Check sheet for the modelled part. Datum: model origin and axes. Units: mm. Face numbers are marked on the shaded views. A direction names the side the tool comes from. Round coordinates to 2 decimals unless told otherwise and drop trailing zeros. Order: outer loops, then holes, each group sorted by start corner. A loop starts at its lowest first (then second) coordinate and runs counter-clockwise, first axis right, second up. Notation, with made-up numbers: (-4, -37) -> (44, -37) arc R23 ccw to (44, -26) -> close; hole circle Ø10 at (-38.75, 66). An arc over 180 degrees is marked (long way). Use CSV: the item, a comma, the result in double quotes.
```python
from build123d import *

# Parameters (mm, degrees)
BOSS_EXTRUDE1_DEPTH = 19.05
SKETCH2_R           = 3
CUT_EXTRUDE1_DEPTH  = 3.175
CUT_EXTRUDE2_REACH  = 48.785
SKETCH3_R           = 3
FILLET1_R           = 10


with BuildPart() as part:
    # Sketch1 → Boss-Extrude1 (new body)
    with BuildSketch(Plane(origin=(0, 0, 0), x_dir=(1, 0, 0), z_dir=(0, 1, 0))):
        Polygon((0, 0), (37.625, 0), (37.625, -6.35), (0, -6.35), (0, -9.525), (40.8, -9.525), (40.8, 3.175), (0, 3.175), align=None)
    extrude(amount=BOSS_EXTRUDE1_DEPTH)

    # Sketch2 → Cut-Extrude1 (cut)
    with BuildSketch(Plane(origin=(40.8, 0, 0), x_dir=(0, 0, -1), z_dir=(1, 0, 0))):
        with Locations((-3.175, 9.525)):
            Circle(SKETCH2_R)
    extrude(amount=-CUT_EXTRUDE1_DEPTH, mode=Mode.SUBTRACT)

    # Cut-Extrude2: up to this face of the body (flat: up to its plane)
    cut_extrude2_end = Plane(part.part.faces().sort_by_distance((20.4, 9.525, -3.175))[0])
    # Sketch3 → Cut-Extrude2 (cut, up to the picked face)
    with BuildSketch(Plane.XY.offset(9.525), mode=Mode.PRIVATE) as cut_extrude2_sk1:
        with Locations((12.7, 9.525)):
            Circle(SKETCH3_R)
    cut_extrude2_tool1 = split(extrude(cut_extrude2_sk1.sketch, amount=-CUT_EXTRUDE2_REACH, mode=Mode.PRIVATE), bisect_by=cut_extrude2_end, keep=Keep.BOTH, mode=Mode.PRIVATE)
    add(cut_extrude2_tool1.solids().sort_by(Axis((12.7, 9.525, 9.525), (0, 0, -1)))[0], mode=Mode.SUBTRACT)

    # Fillet1
    # the kernel refuses this fillet: 10 mm, written as the material it takes off along each edge
    with BuildSketch(Plane(origin=(0, 0, -28.175), x_dir=(0, 1, 0), z_dir=(0, 0, 1)), Plane(origin=(0, 19.05, -18.65), x_dir=(1, 0, 0), z_dir=(0, 0, 1))) as fillet1_piece_1:
        with BuildLine():
            CenterArc((FILLET1_R, -FILLET1_R), FILLET1_R, 90, 90)
            Line((0, -FILLET1_R), (0, 0))
            Line((0, 0), (FILLET1_R, 0))
        make_face()
    extrude(amount=53.175, mode=Mode.SUBTRACT)
    with BuildSketch(Plane(origin=(0, 19.05, -28.175), x_dir=(0, -1, 0), z_dir=(0, 0, 1)), Plane(origin=(0, 0, -18.65), x_dir=(1, 0, 0), z_dir=(0, 0, 1))) as fillet1_piece_2:
        with BuildLine():
            CenterArc((FILLET1_R, FILLET1_R), FILLET1_R, 180, 90)
            Line((0, FILLET1_R), (0, 0))
            Line((0, 0), (FILLET1_R, 0))
        make_face()
    extrude(amount=53.175, mode=Mode.SUBTRACT)


solid = part.part
```
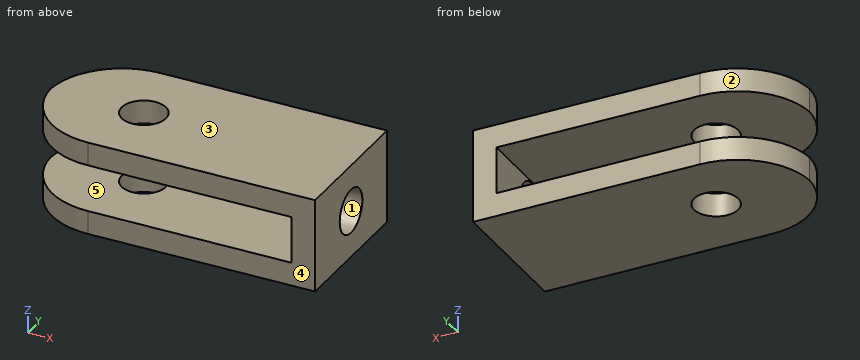
Q1. Sectioned sample at D-D, the plane y = 7.5. Enter the section's corners in (x, z) (3 decimals), then the cut area to 3 significant figures.
Result sheet:
outline,"(0.318, -3.175) -> (10.487, -3.175) -> (10.487, 0) -> (0.318, 0) -> close; (0.318, 6.35) -> (10.487, 6.35) -> (10.487, 9.525) -> (0.318, 9.525) -> close; (14.913, -3.175) -> (40.8, -3.175) -> (40.8, 0.962) -> (37.625, 0.962) -> (37.625, 0) -> (14.913, 0) -> close; (14.913, 6.35) -> (37.625, 6.35) -> (37.625, 5.388) -> (40.8, 5.388) -> (40.8, 9.525) -> (14.913, 9.525) -> close"
area,"235 mm^2"
Q2. Access from +Z, -Z, +X, -X, +Y, -Y to the whole of each face (thin tool, end or side, straight path). Record for the marked faces 4 and 5.
Result sheet:
face 4,"+Z, -Z, +X, -X, -Y"
face 5,"-X, +Y, -Y"
Q3. Scan lines: L1, parallel to Y at x = 12.7, z = -1.3 (3 decimals); L2, parallel to Z at x = 5.5, y = 14 (3 decimals). Record each from-to range of solid material in increasing order.
Result sheet:
L1,"y = 0 to 6.525, 12.525 to 19.05"
L2,"z = -3.175 to 0, 6.35 to 9.525"
Q4. Sectioned sample at B-B, the plane x = 27.5. Enter the section's corners in (y, z) (3 decimals), then the cut area to 3 significant figures.
Result sheet:
outline,"(0, -3.175) -> (19.05, -3.175) -> (19.05, 0) -> (0, 0) -> close; (0, 6.35) -> (19.05, 6.35) -> (19.05, 9.525) -> (0, 9.525) -> close"
area,"121 mm^2"
Q5. Sectioned sample at C-C, the plane z = 4.5. Enter the section's corners in (x, y) (3 decimals).
Result sheet:
outline,"(37.625, 0) -> (40.8, 0) -> (40.8, 6.833) -> (37.625, 6.833) -> close; (37.625, 12.217) -> (40.8, 12.217) -> (40.8, 19.05) -> (37.625, 19.05) -> close"
Q6. Go/stop test with a flat-tipped pin: pin 1 (5.5 mm diameter, centred on x = 12.7, y = 9.525, fed in from -Z). Record where the tip stops, or that it passes through.
Result sheet:
pin 1,"passes through"
Q7. Sectioned sample at A-A, the plane x = 12.7. Enter the section's corners in (y, z) (3 decimals), then the cut area to 3 significant figures.
Result sheet:
outline,"(0, -3.175) -> (6.525, -3.175) -> (6.525, 0) -> (0, 0) -> close; (0, 6.35) -> (6.525, 6.35) -> (6.525, 9.525) -> (0, 9.525) -> close; (12.525, -3.175) -> (19.05, -3.175) -> (19.05, 0) -> (12.525, 0) -> close; (12.525, 6.35) -> (19.05, 6.35) -> (19.05, 9.525) -> (12.525, 9.525) -> close"
area,"82.9 mm^2"
Q8. Mould release check, pull along Z, two halves, no side actions. Record for the marked faces 1, 2 and 3: pulls with the +Z half, pulls with the -Z half, needs draft (parallel to the pull), parting line crosses it, or undercut.
Result sheet:
face 1,"undercut"
face 2,"needs draft"
face 3,"pulls with the +Z half"
